```python
from build123d import *

# Parameters (mm, degrees)
SKETCH1_W           = 45
SKETCH1_H           = 26.5
BOSS_EXTRUDE1_DEPTH = 17
FILLET1_R           = 3
SKETCH2_R           = 3.5
SKETCH2_R_2         = 2.5
BOSS_EXTRUDE2_DEPTH = 1.5


with BuildPart() as part:
    # Sketch1 → Boss-Extrude1 (new body)
    with BuildSketch(Plane(origin=(0, 0, 0), x_dir=(1, 0, 0), z_dir=(0, 1, 0))):
        with Locations((0.552556883, 5.047981579)):
            Rectangle(SKETCH1_W, SKETCH1_H)
    extrude(amount=BOSS_EXTRUDE1_DEPTH)

    # Fillet1
    fillet1_edges = [part.edges().sort_by_distance(p)[0] for p in [
        (0.552556883, 17, -18.297981579),
        (0.552556883, 0, -18.297981579),
        (0.552556883, 0, 8.202018421),
        (0.552556883, 17, 8.202018421),
    ]]
    fillet(fillet1_edges, radius=FILLET1_R)

    # Sketch2 → Boss-Extrude2 (add)
    with BuildSketch(Plane(origin=(23.052556883, 0, 0), x_dir=(0, 0, -1), z_dir=(1, 0, 0))):
        with Locations(Location((11.297981579, 8.5, 0), (0, 0, 180))):
            Circle(SKETCH2_R)
        with Locations(Location((-1.702018421, 8.5, 0), (0, 0, 180))):
            Circle(SKETCH2_R_2)
    extrude(amount=BOSS_EXTRUDE2_DEPTH)


solid = part.part
```
Part model, mm, in its own coordinate system. A direction names the side the tool comes from. Give positions to 0.01 mm unless a question says otherwise; leave off trailing zeros. Order: outer loops, then holes, each group sorted by start corner. A loop starts at its lowest first (then second) coordinate and runs counter-clockwise, first axis right, second up. Notation, with made-up numbers: M -3.75,-15.5 L 54.25,-15.5 A25 ccw 54.25,12.5 Z; hole C 45,33.5 d3. An arc over 180 degrees is marked long. Use a Markdown table: item, result. Add a question column.
(1) Saw through at C-C, the plane y = 8.5. Give the cut face in (x, z).
(2) Saw through at A-A, the plane x = 19. Give the cut face in (y, z).
(3) 3-axis set-ups, long thin cutter, end or side, ignore diameter. For faces 5 (the face through (23.053, 8, -5)), 6 (the face through (24.553, 8, 2)): which of +Z, -Z, +X, -X, +Y, -Y reach the whole face in a straight line?
(4) Saw through at B-B, the plane z = -10.5. Give the cut face in (x, y).
(5) Probe line 1 along X through (y, z) = (4.25, 2); line 2 along Y through (x, z) = (7, 6.25); line 3 along Y through (x, z) = (-8.5, -16.75). List the from-to ranges inside material, lowest first. Write a range as [from, to].
(6) Mould opens along Z. For faces 1 (the face through (0, 8, 8.202)), 2 (the face through (0.87, 16.1, -17.44)), 3 (the face through (23.79, 10.94, 1.16)), 4 (the face through (0, 17, -5)) say: +Z half, -Z half, draft (parallel to the pull), parting line (faces both ways), or undercut.
(7) Saw through at D-D, the plane z = -4.5. Give the cut face in (x, y), and give its area (3 significant figures).
Answer key:
| question | item | result |
|---|---|---|
| 1 | outline | M -21.95,-18.3 L 23.05,-18.3 L 23.05,-14.8 L 24.55,-14.8 L 24.55,-7.8 L 23.05,-7.8 L 23.05,-0.8 L 24.55,-0.8 L 24.55,4.2 L 23.05,4.2 L 23.05,8.2 L -21.95,8.2 Z |
| 2 | outline | M 0,-15.3 A3 ccw 3,-18.3 L 14,-18.3 A3 ccw 17,-15.3 L 17,5.2 A3 ccw 14,8.2 L 3,8.2 A3 ccw 0,5.2 Z |
| 3 | face 5 | +X |
| 3 | face 6 | +Z, -Z, +X, +Y, -Y |
| 4 | outline | M -21.95,0 L 23.05,0 L 23.05,5.09 L 24.55,5.09 L 24.55,11.91 L 23.05,11.91 L 23.05,17 L -21.95,17 Z |
| 5 | line 1 | [-21.95, 23.05] |
| 5 | line 2 | [0.19, 16.81] |
| 5 | line 3 | [0.37, 16.63] |
| 6 | face 1 | +Z half |
| 6 | face 2 | -Z half |
| 6 | face 3 | undercut |
| 6 | face 4 | draft |
| 7 | outline | M -21.95,0 L 23.05,0 L 23.05,17 L -21.95,17 Z |
| 7 | area | 765 mm^2 |
